Here's how the part is built. I have some questions about the finished solid (model axes, mm). Face numbers are marked on the shaded views. A direction names the side the tool comes from. Coordinates: 2 decimals unless noted, no trailing zeros. Write each loop counter-clockwise with the first axis right and the second up, starting at its lowest first coordinate (ties: lowest second). Pieces come first, ordered by that corner, then holes.
(1) Imagine slicing it at C-C, the plane y = 0. State how many separate pieces and enclosed holes the cut face has, plus the area to 3 significant figures.
(2) For pin 1 Ø12 at (x, z) = (57, -3) entering from -Y (3 decimals); pin 2 Ø1 at (x, z) = (29, 5) entering from -Y; pin 3 Ø4 at (y, z) = (-13, -15) entering from -X, each with a flat end and sliding along its axis, tell me the tip position at first contact or that it passes through.
(3) Imagine slicing it at B-B, the plane x = 71.5. List the corners of the cut face in (y, z) for me.
(4) Thinking about a two-plate mould opening in Y: for the marked faces 3, 4 and 5, which applies, released by +Y, released by -Y, zero draft, split by the parting line, or undercut?
(5) Please list where these lines run through material, in increasing order: probe 1 along X at (y, z) = (-5, -0.75); probe 2 along Z at (x, y) = (4.5, -3.5); probe 3 along Y at (x, z) = (34, -1) (3 decimals).
(6) Imagine slicing it at D-D, the plane x = 20.5. List the corners of the cut face in (y, z) for me.
(7) Which directions (+Z, -Z, +X, -X, +Y, -Y) give clear straight access to the entire face, cutting with the end or side of a thin tool? Please do the marked faces 1 and 2.
```python
from build123d import *

# Parameters (mm, degrees)
BOSS_EXTRUDE1_DEPTH = 80
SKETCH2_R           = 2.250000000000002
SKETCH2_R_2         = 2.249999999999999
CUT_EXTRUDE1_DEPTH  = 86.91559811815314
SKETCH3_W           = 8.000000000000007
SKETCH3_H           = 15.000000000000002
BOSS_EXTRUDE2_DEPTH = 5
CHAMFER1_SIZE       = 8
FILLET1_R           = 1
BOSS_EXTRUDE3_DEPTH = 7
BOSS_EXTRUDE4_START = 2.5
BOSS_EXTRUDE4_DEPTH = 2.5
FILLET3_R           = 1


with BuildPart() as part:
    # Sketch1 → Boss-Extrude1 (new body)
    with BuildSketch(Plane.YZ):
        Polygon((-22.5, -17.5), (-7.500000000000001, 2.5000000000000004), (-7.499999999999999, -2.4999999999999996), (-20.099999999999994, -19.300000000000004), align=None)
        Polygon((7.500000000000001, 2.5000000000000004), (7.500000000000001, -2.4999999999999996), (-7.499999999999999, -2.4999999999999996), (-7.500000000000001, 2.5000000000000004), align=None)
        Polygon((7.500000000000001, 2.5000000000000004), (7.500000000000001, -2.4999999999999996), (20.099999999999994, -19.300000000000004), (22.5, -17.5), align=None)
    extrude(amount=BOSS_EXTRUDE1_DEPTH)

    # Sketch2 → Cut-Extrude1 (cut, through all)
    with BuildSketch(Plane.XY.offset(2.5000000000000004)):
        with Locations((5.5, 0)):
            Circle(SKETCH2_R)
        with Locations((15.5, 0)):
            Circle(SKETCH2_R_2)
        Polygon((80, 7.0000000000000036), (30.5, 6.999999999999997), (30.5, -7.000000000000003), (80, -6.9999999999999964), align=None)
    extrude(amount=-CUT_EXTRUDE1_DEPTH, mode=Mode.SUBTRACT)

    # Sketch3 → Boss-Extrude2 (add)
    with BuildSketch(Plane.XY.offset(2.5000000000000004)):
        with Locations((26.47757310370073, 0)):
            Rectangle(SKETCH3_W, SKETCH3_H)
    extrude(amount=BOSS_EXTRUDE2_DEPTH)

    # Chamfer1
    # the kernel refuses this chamfer: 8 mm, written as the material it takes off along each edge
    with BuildSketch(Plane(origin=(22.477573103700728, 28.073463903727287, 7.5), x_dir=(-0.027495876610586494, 0, -0.9996219169112968), z_dir=(0, -1, 0))) as chamfer1_piece_1_section:
        Polygon((CHAMFER1_SIZE * 0.999621916911, CHAMFER1_SIZE * 0.0274958766106), (-CHAMFER1_SIZE * 0.0274958766106, CHAMFER1_SIZE * 0.999621916911), (0, 0), align=None)
    chamfer1_piece_1 = extrude(amount=56.146927807454574, mode=Mode.PRIVATE)
    chamfer1_piece_1 = split(chamfer1_piece_1, bisect_by=Plane(origin=(25.44368954303125, 0, 2.5000000000000004), z_dir=(0, 0, 1)), keep=Keep.TOP, mode=Mode.PRIVATE)
    add(chamfer1_piece_1, mode=Mode.SUBTRACT)

    # Fillet1
    fillet1_edges = [part.edges().sort_by_distance(p)[0] for p in [
        (40, -7.499999999999999, -2.4999999999999996),
        (40, 7.500000000000001, -2.4999999999999996),
        (27.977573103699285, 7.500000000000001, 2.5000000000000004),
        (27.977573103699285, -7.500000000000001, 2.5000000000000004),
        (30.47757310370073, 0, 7.5),
    ]]
    fillet(fillet1_edges, radius=FILLET1_R)

    # Sketch4 → Boss-Extrude3 (add)
    with BuildSketch(Plane(origin=(0, 0, 0), x_dir=(0, -1, 0), z_dir=(-1, 0, 0))):
        with BuildLine():
            Line((22.5, -17.5), (7.500000000000001, 2.5000000000000004))
            Line((7.500000000000001, 2.5000000000000004), (-7.500000000000001, 2.5000000000000004))
            Line((-7.500000000000001, 2.5000000000000004), (-22.5, -17.5))
            Line((-22.5, -17.5), (-20.099999999999994, -19.300000000000004))
            Line((-20.099999999999994, -19.300000000000004), (-7.800000000000002, -2.9000000000000004))
            ThreePointArc((-7.800000000000002, -2.9000000000000004), (-7.447213595499958, -2.6055728090000834), (-6.999999999999999, -2.4999999999999987))
            Line((-6.999999999999999, -2.4999999999999987), (6.999999999999998, -2.4999999999999996))
            ThreePointArc((6.999999999999998, -2.4999999999999996), (7.4472135954999565, -2.6055728090000834), (7.799999999999999, -2.8999999999999995))
            Line((7.799999999999999, -2.8999999999999995), (20.099999999999998, -19.300000000000008))
            Line((20.099999999999998, -19.300000000000008), (22.5, -17.5))
        make_face()
    extrude(amount=BOSS_EXTRUDE3_DEPTH)

    # Sketch6 → Boss-Extrude4 (add)
    with BuildSketch(Plane.YZ.offset(80).offset(BOSS_EXTRUDE4_START)):
        with BuildLine():
            Line((-6.9999999999999964, -2.4999999999999987), (-6.9999999999999964, 2.5000000000000004))
            Line((-6.9999999999999964, 2.5000000000000004), (7.0000000000000036, 2.5000000000000004))
            Line((7.0000000000000036, 2.5000000000000004), (7.0000000000000036, -2.4999999999999996))
            ThreePointArc((7.0000000000000036, -2.4999999999999996), (7.44721359549996, -2.605572809000085), (7.800000000000002, -2.9000000000000004))
            Line((7.800000000000002, -2.9000000000000004), (20.099999999999994, -19.300000000000004))
            Line((20.099999999999994, -19.300000000000004), (-20.099999999999998, -19.300000000000008))
            Line((-20.099999999999998, -19.300000000000008), (-7.799999999999999, -2.8999999999999995))
            ThreePointArc((-7.799999999999999, -2.8999999999999995), (-7.447213595499956, -2.6055728090000825), (-6.9999999999999964, -2.4999999999999987))
        make_face()
        with BuildLine():
            ThreePointArc((-6.9999999999999964, -2.4999999999999987), (-7.447213595499956, -2.6055728090000825), (-7.799999999999999, -2.8999999999999995))
            Line((-7.799999999999999, -2.8999999999999995), (-20.099999999999998, -19.300000000000008))
            Line((-20.099999999999998, -19.300000000000008), (-22.5, -17.5))
            Line((-22.5, -17.5), (-7.500000000000001, 2.5000000000000004))
            Line((-7.500000000000001, 2.5000000000000004), (-6.9999999999999964, 2.5000000000000004))
            Line((-6.9999999999999964, 2.5000000000000004), (-6.9999999999999964, -2.4999999999999987))
        make_face()
        with BuildLine():
            Line((7.500000000000001, 2.5000000000000004), (7.0000000000000036, 2.5000000000000004))
            Line((7.0000000000000036, 2.5000000000000004), (7.0000000000000036, -2.4999999999999996))
            ThreePointArc((7.0000000000000036, -2.4999999999999996), (7.44721359549996, -2.605572809000085), (7.800000000000002, -2.9000000000000004))
            Line((7.800000000000002, -2.9000000000000004), (20.099999999999994, -19.300000000000004))
            Line((20.099999999999994, -19.300000000000004), (22.5, -17.5))
            Line((22.5, -17.5), (7.500000000000001, 2.5000000000000004))
        make_face()
    extrude(amount=-BOSS_EXTRUDE4_DEPTH)

    # Fillet3
    fillet3_edges = [part.edges().sort_by_distance(p)[0] for p in [
        (-7, -21.299999999999997, -18.400000000000002),
        (-7, -15, -7.5),
        (-7, 0, 2.5000000000000004),
        (37.75, 22.5, -17.5),
        (-7, 15, -7.5),
        (-7, 21.299999999999997, -18.400000000000002),
        (-7, 13.949999999999998, -11.100000000000001),
        (-7, 7.447213595499958, -2.605572809000084),
        (-7, 8.9e-16, -2.499999999999999),
        (-7, -7.4472135954999565, -2.6055728090000834),
        (-7, -13.95, -11.100000000000005),
        (37.75, -22.5, -17.5),
        (82.5, 0, 2.5000000000000004),
        (82.5, -15, -7.5),
        (82.5, -21.299999999999997, -18.400000000000002),
        (82.5, 0, -19.300000000000004),
        (82.5, 21.299999999999997, -18.400000000000002),
        (82.5, 15, -7.5),
    ]]
    fillet(fillet3_edges, radius=FILLET3_R)


solid = part.part
```
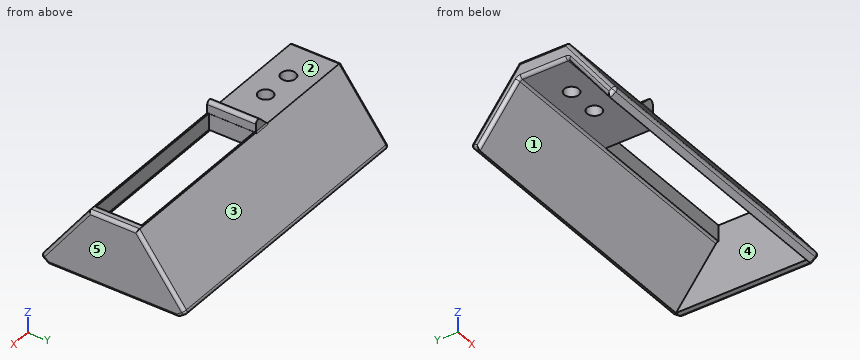
Recorded:
1. separate pieces: 4
1. enclosed holes: 0
1. area: 207 mm2
2. pin 1: stops at y = -16.125
2. pin 2: stops at y = -7.5
2. pin 3: stops at x = 80
3. outline: (-21.9, -16.7) arc R1 ccw to (-21.7, -18.1) - (-20.1, -19.3) - (-7.8, -2.9) arc R1 cw to (-7, -2.5) - (-7, 2.5) - (-7.5, 2.5) - close; (7, -2.5) arc R1 cw to (7.8, -2.9) - (20.1, -19.3) - (21.7, -18.1) arc R1 ccw to (21.9, -16.7) - (7.5, 2.5) - (7, 2.5) - close
4. face 3: released by +Y
4. face 4: undercut
4. face 5: zero draft
5. probe 1: x = -7 to 30.5, 80 to 82.5
5. probe 2: z = -2.5 to 2.5
5. probe 3: y = -10.125 to -7, 7 to 10.125
6. outline: (-21.9, -16.7) arc R1 ccw to (-21.7, -18.1) - (-20.1, -19.3) - (-7.8, -2.9) arc R1 cw to (-7, -2.5) - (7, -2.5) arc R1 cw to (7.8, -2.9) - (20.1, -19.3) - (21.7, -18.1) arc R1 ccw to (21.9, -16.7) - (7.5, 2.5) - (-7.5, 2.5) - close
7. face 1: -Z, -X
7. face 2: +Z, -X, +Y, -Y
